Autodesk Inventor part; units mm, degrees
ref_plane "Work Plane1" through (0, 2.59, 0) normal (0, -1, 0) x (1, 0, 0)
ref_plane "YZ Plane" through (0, 0, 0) normal (1, 0, 0) x (0, 1, 0)
ref_plane "XZ Plane" through (0, 0, 0) normal (0, 1, 0) x (-1, 0, 0)
sketch "Sketch1" plane through (0, 0, 0) normal (0, 1, 0) x (-1, 0, 0)
  line L0 (10.41, 7.935) -> (-10.41, 7.935)
  line L1 (-10.41, 7.935) -> (-10.41, -7.935)
  line L2 (-10.41, -7.935) -> (10.41, -7.935)
  line L3 (10.41, -7.935) -> (10.41, 7.935)
  point P0 (0, 0)
  dimension "d0" = 15.87
  dimension "d1" = 7.935
  dimension "d2" = 20.82
  dimension "d3" = 10.41
extrude "Extrusion1" add sketch "Sketch1" along normal blind 5.31
chamfer "Chamfer1" distance 2.72 angle 15 1 edges at (0, 5.31, 7.935) measured on face at (-3.47, 1.77, 7.935)
chamfer "Chamfer2" distance 2.72 angle 15 1 edges at (10.41, 5.31, -0.3644) measured on face at (10.41, 3.54, -2.8879)
chamfer "Chamfer3" distance 2.72 angle 15 1 edges at (-0.3644, 5.31, -7.935) measured on face at (3.2271, 1.77, -7.935)
chamfer "Chamfer4" distance 2.72 angle 15 1 edges at (-10.41, 5.31, 0) measured on face at (-10.41, 3.4967, -2.4021)
sketch "Sketch3" plane through (0, 0, 0) normal (0, -1, 0) x (1, 0, 0)
  line L0 (-9.11, 6.86) -> (3.97, 6.86)
  line L1 (3.97, 6.86) -> (3.97, -6.86)
  line L2 (3.97, -6.86) -> (-9.11, -6.86)
  line L3 (-9.11, -6.86) -> (-9.11, 6.86)
  line L4 (-10.41, -7.935) -> (-10.41, 7.935)
  point P0 (0, 0)
  dimension "d20" = 13.08
  dimension "d21" = 13.72
  dimension "d22" = 6.86
  dimension "d23" = 1.3
extrude "Extrusion2" add sketch "Sketch3" along normal blind 0.01
sketch "Sketch2" plane through (0, 5.31, 0) normal (0, 1, 0) x (1, 0, 0)
  circle A0 centre (-4.9, 0) radius 1.83
  line L0 (-10.41, 7.935) -> (-10.41, -7.935)
  point P0 (0, 0)
  dimension "d18" = 5.51
  dimension "d19" = 3.66
extrude "Extrusion3" cut sketch "Sketch2" against normal through all
sketch "Sketch4" plane through (0, 5.31, 0) normal (0, 1, 0) x (1, 0, 0)
  line L0 (-10.41, 7.935) -> (-10.41, -7.935)
  line L1 (-10.41, -7.935) -> (10.41, -7.935)
  line L2 (-9.3708, -7.935) -> (-0.6355, -7.935)
  circle A0 centre (-4.72, -7.935) radius 2.745
  point P0 (0, 0)
  dimension "d30" = 5.49
  dimension "d31" = 5.69
extrude "Extrusion4" cut sketch "Sketch4" against normal blind 3.14
mirror "Mirror1" about plane through (0, 0, 0) normal (0, 0, 1) of "Extrusion4"
chamfer "Chamfer5" distance 1 angle 45 3 edges at (-4.72, 5.31, 5.19) (-6.73, 5.31, 0) (-4.72, 5.31, -5.19)
ref_plane "Work Plane1" through (0, 2.59, 0) normal (0, -1, 0) x (1, 0, 0)
sketch "Sketch5" plane through (0, 2.59, 0) normal (0, -1, 0) x (1, 0, 0)
  line L0 (9.0645, 1.715) -> (14.7, 1.715)
  line L1 (14.7, 1.715) -> (14.7, -1.715)
  line L2 (14.7, -1.715) -> (9.0645, -1.715)
  line L3 (9.0645, -1.715) -> (9.0645, 1.715)
  line L4 (10.41, 7.935) -> (10.41, -7.935)
  line L5 (10.41, 0) -> (13.4225, 0)
  line L6 (10.1151, 6.655) -> (14.7, 6.655)
  line L7 (14.7, 6.655) -> (14.7, 4.265)
  line L8 (14.7, 4.265) -> (10.1151, 4.265)
  line L9 (10.1151, 4.265) -> (10.1151, 6.655)
  line L10 (14.7, 5.46) -> (14.8506, 5.46)
  line L11 (14.7, 6.16) -> (14.4142, 6.655)
  line L12 (14.7, 4.76) -> (14.4142, 4.265)
  line L13 (14.7, 0.7) -> (14.114, 1.715)
  line L14 (14.7, -0.7) -> (14.114, -1.715)
  line L15 (10.1151, -6.655) -> (14.7, -6.655)
  line L16 (14.7, -6.655) -> (14.7, -4.265)
  line L17 (14.7, -4.265) -> (10.1151, -4.265)
  line L18 (10.1151, -4.265) -> (10.1151, -6.655)
  line L19 (14.7, -6.16) -> (14.4142, -6.655)
  line L20 (14.7, -4.76) -> (14.4142, -4.265)
  point P0 (0, 0)
  dimension "d38" = 3.43
  dimension "d39" = 1.715
  dimension "d40" = 4.29
  dimension "d41" = 0
  dimension "d42" = 2.39
  dimension "d43" = 5.46
  dimension "d44" = 1.4
  dimension "d45" = 0.7
  dimension "d46" = 1.4
  dimension "d47" = 0.7
  dimension "d48" = 30
  dimension "d49" = 30
  dimension "d50" = 30
  dimension "d51" = 30
extrude "Extrusion5" add sketch "Sketch5" against normal blind 0.86 contours L17 L20 L16 L19 L15 L4 | L4 L15 L18 L17 | L8 L9 L6 L4 | L4 L6 L11 L7 L12 L8 | L13 L1 L14 L2 L4 L0 | L4 L2 L3 L0
sketch "Sketch6" plane through (14.7, 2.59, 0.7) normal (1, 0, 0) x (0, 0, -1)
  line L0 (-5.46, 0) -> (-5.46, 0.86)
  line L1 (-4.06, 0) -> (-4.06, 0.86)
  line L2 (-5.46, 0) -> (-4.06, 0)
  line L3 (-4.06, 0) -> (-4.06, 0.86)
  line L4 (-4.06, 0.86) -> (-5.46, 0.86)
  line L5 (-5.46, 0.86) -> (-5.46, 0)
  line L6 (0, 0) -> (0, 0.86)
  line L7 (1.4, 0) -> (1.4, 0.86)
  line L8 (0, 0) -> (1.4, 0)
  line L9 (1.4, 0) -> (1.4, 0.86)
  line L10 (1.4, 0.86) -> (0, 0.86)
  line L11 (0, 0.86) -> (0, 0)
  line L12 (5.46, 0) -> (5.46, 0.86)
  line L13 (4.965, 0.86) -> (7.355, 0.86)
  line L14 (5.46, 0) -> (6.86, 0)
  line L15 (6.86, 0) -> (6.86, 0.86)
  line L16 (6.86, 0.86) -> (5.46, 0.86)
  line L17 (5.46, 0.86) -> (5.46, 0)
  point P0 (0.7, -2.59)
  dimension "d54" = 1.4
sketch "Sketch7" plane through (0, 0, 0) normal (0, 0, 1) x (1, 0, 0)
  line L0 (14.7, 2.59) -> (14.7, 3.45)
  line L1 (14.7, 3.02) -> (15.6, 3.02)
  line L2 (18.3, 5.72) -> (18.3, 8.36)
  line L3 (10.41, 0) -> (-10.41, 0)
  arc A0 (15.6, 3.02) -> (18.3, 5.72) centre (15.6, 5.72) ccw
  point P0 (0, 0)
  point P1 (18.3, 3.02)
  dimension "d55" = 8.36
  dimension "d56" = 3.6
  dimension "d57" = 2.7
sweep "Sweep1" add profiles "Sketch6" path "Sketch7" path curves L1 A0 L2
properties part number "TO-247-Underheat"
Geometry: final body of the model. Coordinates: model frame, mm. A direction names the side the tool comes from. Coordinates: 2 decimals unless noted, no trailing zeros. Loops run counter-clockwise (first coordinate to the right, second up) from the corner with the lowest first, then second, coordinate; pieces in that order, holes last. Notation, with made-up numbers: (29, 77.5) -> (41, 77.5) arc R22 ccw to (41, 108.5) -> close; hole circle Ø9 at (-11, 62). An arc over 180 degrees is marked (long way). Use a Markdown table: item, result. Add a question column.
(1) Section query D-D, the plane y = 4. Return loops of the section in (x, z) (3 decimals).
(2) Mould query, pull axis Z, two halves, no side actions, for faces 1 (the flat face through (12, 3, 1.715)), 2 (the flat face through (-10.41, 1, 0)), 3 (the conical face through (-4.8, 4.5, -5)). Classes: pulls with the +Z half, pulls with the -Z half, needs draft (parallel to the pull), parting line crosses it, or undercut.
(3) Section query C-C, the plane y = 7.75. Return loops of the section in (x, z).
(4) Section query A-A, the plane x = 12.25. Return loops of the section in (y, z) (3 decimals).
(5) Line query: line 1 along Z through (x, y) = (-4.9, 1.55) (3 decimals); line 2 along X through (y, z) = (2.1, 0); line 3 along Y through (x, z) = (3.5, 1.5). Output: solid intervals per line, ascending.
(6) Pin query (flat end, axial travel): pin 1 Ø4 at (x, y) = (-2.5, 4.5) entering from -Z (3 decimals); pin 2 Ø2 at (x, z) = (-5.5, -7) entering from +Y; pin 3 Ø5 at (y, z) = (7, 1.5) entering from -X; pin 4 Ø3 at (x, z) = (-5.5, 6) entering from +Y. Return the tip coordinate at first contact, or that it passes through.
(7) Access query for faces 4 (the flat face through (14.41, 3.01, 1.2)), 5 (the flat face through (17.87, 7, 0)), 6 (the flat face through (12, 2.59, 0)), 7 (the flat face through (-5, 2.17, 7)), 8 (the flat face through (13, 3.45, -5)). Directions: +Z, -Z, +X, -X, +Y, -Y. A direction counts if a zero-diameter tool reaches every point of the face in a straight line with its end or side. Return the directions, or none.
Answer:
| question | item | result |
|---|---|---|
| 1 | outline | (-10.032, -7.557) -> (-7.439, -7.557) arc R2.745 cw to (-2.001, -7.557) -> (10.032, -7.557) -> (10.032, 7.557) -> (-2.001, 7.557) arc R2.745 cw to (-7.439, 7.557) -> (-10.032, 7.557) -> close; (17.081, -6.16) -> (18.215, -6.16) -> (18.215, -4.76) -> (17.081, -4.76) -> close; (17.081, -0.7) -> (18.215, -0.7) -> (18.215, 0.7) -> (17.081, 0.7) -> close; (17.081, 4.76) -> (18.215, 4.76) -> (18.215, 6.16) -> (17.081, 6.16) -> close; hole circle Ø3.66 at (-4.9, 0) |
| 2 | face 1 | undercut |
| 2 | face 2 | needs draft |
| 2 | face 3 | pulls with the -Z half |
| 3 | outline | (17.87, -6.16) -> (18.73, -6.16) -> (18.73, -4.76) -> (17.87, -4.76) -> close; (17.87, -0.7) -> (18.73, -0.7) -> (18.73, 0.7) -> (17.87, 0.7) -> close; (17.87, 4.76) -> (18.73, 4.76) -> (18.73, 6.16) -> (17.87, 6.16) -> close |
| 4 | outline | (2.59, -6.655) -> (3.45, -6.655) -> (3.45, -4.265) -> (2.59, -4.265) -> close; (2.59, -1.715) -> (3.45, -1.715) -> (3.45, 1.715) -> (2.59, 1.715) -> close; (2.59, 4.265) -> (3.45, 4.265) -> (3.45, 6.655) -> (2.59, 6.655) -> close |
| 5 | line 1 | z = -7.935 to -1.83, 1.83 to 7.935 |
| 5 | line 2 | x = -10.41 to -6.73, -3.07 to 10.41 |
| 5 | line 3 | y = -0.01 to 5.31 |
| 6 | pin 1 | stops at z = -7.935 |
| 6 | pin 2 | stops at y = 2.17 |
| 6 | pin 3 | stops at x = -9.9 |
| 6 | pin 4 | stops at y = 5.15 |
| 7 | face 4 | +X, +Y, -Y |
| 7 | face 5 | +Z, -Z, -X, +Y |
| 7 | face 6 | +Z, -Z, +X, -Y |
| 7 | face 7 | +Z, +Y |
| 7 | face 8 | +Z, -Z, +Y |
